Geometry check sheet. Reference: the model listing, model coordinates, mm. A direction names the side the tool comes from. Give positions to 0.01 mm unless a question says otherwise; leave off trailing zeros. Loops run counter-clockwise (first coordinate to the right, second up) from the corner with the lowest first, then second, coordinate; pieces in that order, holes last. Notation, with made-up numbers: (65, -34.75) - (78, -34.75) arc R26 cw to (78, 0.25) - close; hole circle Ø6 at (1, -27). An arc over 180 degrees is marked (long way). One line per question, with ' | ' between items. Start each with the question number.
Autodesk Inventor part; units mm, degrees
ref_plane "YZ Plane" through (0, 0, 0) normal (1, 0, 0) x (0, 1, 0)
ref_plane "XZ Plane" through (0, 0, 0) normal (0, 1, 0) x (-1, 0, 0)
ref_plane "XY Plane" through (0, 0, 0) normal (0, 0, 1) x (1, 0, 0)
sketch "Sketch1" plane through (0, 0, 0) normal (1, 0, 0) x (0, 1, 0)
  line L0 (0, 12.65) -> (0, -12.65) construction
  line L1 (3, 0) -> (3, 1.5)
  line L2 (3, 1.5) -> (2.25, 1.5)
  line L3 (1.75, 2) -> (1.75, 7)
  line L4 (1.75, 7) -> (2.375, 7)
  line L5 (2.375, 7) -> (1.8, 12.65)
  line L6 (1.8, 12.65) -> (0.875, 12.65)
  line L7 (0.875, 12.65) -> (0.875, 0)
  line L8 (3, 0) -> (-3, 0) construction
  line L9 (3, 0) -> (3, -1.5)
  line L10 (3, -1.5) -> (2.25, -1.5)
  line L11 (1.75, -2) -> (1.75, -7)
  line L12 (1.75, -7) -> (2.375, -7)
  line L13 (2.375, -7) -> (1.8, -12.65)
  line L14 (1.8, -12.65) -> (0.875, -12.65)
  line L15 (0.875, -12.65) -> (0.875, 0)
  line L16 (2.25, 1.5) -> (1.75, 2)
  line L17 (2.25, -1.5) -> (1.75, -2)
  point P0 (0, 0)
  point P1 (1.75, 1.5)
  point P2 (1.75, -1.5)
  dimension "d0" = 25.3
  dimension "d1" = 3
  dimension "d2" = 1.5
  dimension "d3" = 6
  dimension "d4" = 3.5
  dimension "d5" = 5.5
  dimension "d6" = 4.75
  dimension "d7" = 3.6
  dimension "d8" = 1.75
  dimension "d9" = 6
  dimension "d10" = 0.5
  dimension "d11" = 0.5
  dimension "d12" = 0.5
  dimension "d13" = 0.5
revolve "Revolution1" add sketch "Sketch1" angle 360 about axis through (0, 0, 12.65) along (0, 0, -1)
properties part number "Adafruit_4764"
(1) Depth check by flat-ended pin: pin 1 Ø1.5 at (x, y) = (-0.5, -0.5) entering from +Z; pin 2 Ø2 at (y, z) = (0.5, 9.5) entering from +X. Enter the tip coordinate at first touch or a pass-through.
(2) Material ranges on line 1 (X direction, y = 0, z = -6.5) (3 decimals); line 2 (X direction, y = 0, z = 1) (3 decimals); line 3 (Z direction, x = -1.2, y = 2.6), recorded low to high.
(3) Section check A-A, the plane x = 0. Record the boundary of the cut face in (y, z) (3 decimals), and give its area (3 significant figures).
(4) Section check C-C, the plane z = -5.75. Record the boundary of the cut face in (x, y) (3 decimals).
(5) Section check D-D, the plane z = 8. Record the boundary of the cut face in (x, y) (3 decimals).
(6) Tool access check on faces 4 (the face through (-0.67, 1.617, -4.535)), 5 (the face through (-0.8, 1.93, 9.79)). Record the directions out of +Z, -Z, +X, -X, +Y, -Y that give a thin tool (end or side, any length) a straight path to the whole face; none if there is none.
(7) Mould release check, pull along Z, two halves, no side actions. Record for faces 1 (the face through (-2, 0, -7)), 2 (the face through (0, -3, 0)), 3 (the face through (0.8, 1.93, -9.79)): pulls with the +Z half, pulls with the -Z half, needs draft (parallel to the pull), parting line crosses it, or undercut.
Numbers:
1) pin 1: z = 12.65 | pin 2: x = 2.21
2) line 1: -1.75 to -0.875, 0.875 to 1.75 | line 2: -3 to -0.875, 0.875 to 3 | line 3: -1.5 to 1.5
3) outline: (-3, -1.5) - (-2.25, -1.5) - (-1.75, -2) - (-1.75, -7) - (-2.375, -7) - (-1.8, -12.65) - (-0.875, -12.65) - (-0.875, 12.65) - (-1.8, 12.65) - (-2.375, 7) - (-1.75, 7) - (-1.75, 2) - (-2.25, 1.5) - (-3, 1.5) - close; (0.875, -12.65) - (1.8, -12.65) - (2.375, -7) - (1.75, -7) - (1.75, -2) - (2.25, -1.5) - (3, -1.5) - (3, 1.5) - (2.25, 1.5) - (1.75, 2) - (1.75, 7) - (2.375, 7) - (1.8, 12.65) - (0.875, 12.65) - close | area: 59.9 mm^2
4) outline: circle Ø3.5 at (0, 0); hole circle Ø1.75 at (0, 0)
5) outline: circle Ø4.546 at (0, 0); hole circle Ø1.75 at (0, 0)
6) face 4: none | face 5: +Z
7) face 1: undercut | face 2: needs draft | face 3: pulls with the -Z half
